```python
from build123d import *

# Parameters (mm, degrees)
BOSS_EXTRUDE1_DEPTH   = 6
M3X0_5_TAPPED_HOLE1_D = 2.5
FILLET1_R             = 1
FILLET2_R             = 2
FILLET3_R             = 1
FILLET4_R             = 2.25
FILLET5_R             = 2.25


with BuildPart() as part:
    # Sketch1 → Boss-Extrude1 (new body)
    with BuildSketch(Plane.XY):
        Polygon((-5.15, 1.75), (-2.575, 1.75), (-2.575, 2.75), (2.575, 2.75), (2.575, 1.75), (5.15, 1.75), (5.15, 0), (2.575, -1.75), (-2.575, -1.75), (-5.15, 0), align=None)
    extrude(amount=BOSS_EXTRUDE1_DEPTH)

    # M3x0.5 Tapped Hole1 (through all)
    with Locations(Plane(origin=(0, 2.75, 0), x_dir=(1, 0, 0), z_dir=(0, 1, 0))):
        with Locations((0, -3)):
            Hole(M3X0_5_TAPPED_HOLE1_D / 2)

    # Fillet1
    fillet1_edges = [part.edges().sort_by_distance(p)[0] for p in [
        (-5.15, 0.875, 0),
    ]]
    fillet(fillet1_edges, radius=FILLET1_R)

    # Fillet2
    fillet2_edges = [part.edges().sort_by_distance(p)[0] for p in [
        (-5.15, 0.875, 6),
    ]]
    fillet(fillet2_edges, radius=FILLET2_R)

    # Fillet3
    fillet3_edges = [part.edges().sort_by_distance(p)[0] for p in [
        (5.15, 0.875, 6),
    ]]
    fillet(fillet3_edges, radius=FILLET3_R)

    # Fillet4
    fillet4_edges = [part.edges().sort_by_distance(p)[0] for p in [
        (5.15, 0.875, 0),
    ]]
    fillet(fillet4_edges, radius=FILLET4_R)

    # Fillet5
    fillet5_edges = [part.edges().sort_by_distance(p)[0] for p in [
        (-2.575, 2.25, 0),
        (2.575, 2.25, 6),
    ]]
    fillet(fillet5_edges, radius=FILLET5_R)


solid = part.part
```
For this review, take the finished solid that the model builds, in its own axes (mm). A direction names the side the tool comes from. Coordinates: 2 decimals unless noted, no trailing zeros. Order: outer loops, then holes, each group sorted by start corner. A loop starts at its lowest first (then second) coordinate and runs counter-clockwise, first axis right, second up. Notation, with made-up numbers: (10, 75.5) - (63, 75.5) arc R28 cw to (63, 112.5) - close; hole circle Ø11 at (-3.75, 8.5). An arc over 180 degrees is marked (long way). Answer as a JSON object with one key per item and string values. Group by question number.
1. We need section A-A on y = 1.4. State the section outline as (x, z) points, then the cut area to 3 significant figures.
2. Clearance check with flat-ended pins moving along their axes: P1, Ø0.5, axis at y = 2.5, z = 4, coming from the -X side (3 decimals); P2, Ø2, axis at y = -1, z = 1, coming from the +X side. State where each tip first meets the part, or that it passes through.
3. For probe 1 along X at (y, z) = (0.5, 2.95); probe 2 along Z at (x, y) = (0, 0.75); probe 3 along X at (y, z) = (-1.4, 2.25), list the stretches that pass through material, from the lowest coordinate up.
4. The part is to be moulded in two halves that separate along Z. For faces 6 (the cylindrical face through (4.21, 0.45, 0.42)), 7 (the cylindrical face through (0.16, 0.47, 1.76)), 8 (the flat face through (-3.84, -0.89, 2.96)), say which applies: pulls with the +Z half, pulls with the -Z half, needs draft (parallel to the pull), parting line crosses it, or undercut.
5. For faces 1 (the flat face through (-2.575, 2, 4)), 2 (the flat face through (2.575, 2, 2)), 3 (the cylindrical face through (4.849, 0.788, 5.715)), 4 (the cylindrical face through (-1.898, 2.257, 0.642)), 5 (the cylindrical face through (1.898, 2.243, 5.358)), list the 3-axis set-ups (+Z, -Z, +X, -X, +Y, -Y) from which the entire face can be reached by the end or side of a thin tool; tool diameter is ignored.
6. We need section D-D on z = 0.4. State the section outline as (x, y) points (3 decimals).
7. We need section C-C on x = 0. State the section outline as (y, z) points.
8. We need section B-B on z = 3. State the section outline as (x, y) points (3 decimals).
Final values:
{
 "1": {"outline": "(-5.15, 1) arc R1 ccw to (-4.15, 0) - (2.9, 0) arc R2.25 ccw to (5.15, 2.25) - (5.15, 5) arc R1 ccw to (4.15, 6) - (-3.15, 6) arc R2 ccw to (-5.15, 4) - close; hole circle Ø2.5 at (0, 3)", "area": "54.5 mm²"},
 "2": {"P1": "x = -2.575", "P2": "x = 5"},
 "3": {"probe 1": "-5.15 to -1.25, 1.25 to 5.15", "probe 2": "0 to 1.75, 4.25 to 6", "probe 3": "-3.09 to -1, 1 to 3.09"},
 "4": {"face 6": "pulls with the -Z half", "face 7": "undercut", "face 8": "needs draft"},
 "5": {"face 1": "+Z, -Z, -X, +Y", "face 2": "+Z, -Z, +X, +Y", "face 3": "+Z, +X, +Y, -Y", "face 4": "-Z, -X, +Y", "face 5": "+Z, +X, +Y"},
 "6": {"outline": "(-4.95, -0.136) - (-2.575, -1.75) - (2.575, -1.75) - (4.181, -0.659) - (4.181, 1.75) - (2.575, 1.75) - (2.575, 2.75) - (-1.606, 2.75) - (-1.606, 1.75) - (-4.95, 1.75) - close"},
 "7": {"outline": "(-1.75, 0) - (2.75, 0) - (2.75, 1.75) - (-1.75, 1.75) - close; (-1.75, 4.25) - (2.75, 4.25) - (2.75, 6) - (-1.75, 6) - close"},
 "8": {"outline": "(-5.15, 0) - (-2.575, -1.75) - (-1.25, -1.75) - (-1.25, 2.75) - (-2.575, 2.75) - (-2.575, 1.75) - (-5.15, 1.75) - close; (1.25, -1.75) - (2.575, -1.75) - (5.15, 0) - (5.15, 1.75) - (2.575, 1.75) - (2.575, 2.75) - (1.25, 2.75) - close"}
}
